Model file for the job. Use its own axes, mm. Face numbers are marked on the shaded views. Round coordinates to 2 decimals unless told otherwise and drop trailing zeros. Order: outer loops, then holes, each group sorted by start corner. A loop starts at its lowest first (then second) coordinate and runs counter-clockwise, first axis right, second up. Notation, with made-up numbers: (-2.75, -21) -> (23.25, -21) arc R21 cw to (23.25, 14) -> close; hole circle Ø10 at (-38.75, -16.75). An arc over 180 degrees is marked (long way). Use CSV: the item, a comma, the result in double quotes.
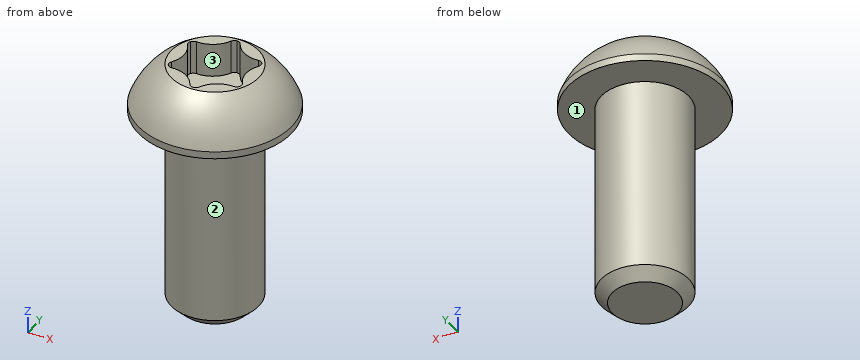
```python
from build123d import *

# Parameters (mm, degrees)
SKETCH12_W         = 14
SKETCH12_H         = 3
CUT_EXTRUDE4_DEPTH = 2.31
CIRPATTERN1_COUNT  = 6
CHAMFER1_SIZE      = 0.75


with BuildPart() as part:
    # Sketch12 → Revolve1 (revolve)
    with BuildSketch(Plane(origin=(0, 0, 0), x_dir=(0, 0, -1), z_dir=(1, 0, 0))):
        with Locations((0, 1.5)):
            Rectangle(SKETCH12_W, SKETCH12_H)
    revolve(axis=Axis((0, 0, -7), (0, 0, 1)))

    # Sketch7 → Revolve2 (revolve)
    with BuildSketch(Plane(origin=(0, 0, 0), x_dir=(0, 0, -1), z_dir=(1, 0, 0)), mode=Mode.PRIVATE) as revolve2_sk:
        with BuildLine():
            Line((-7.495, 5.25), (-7, 5.25))
            Line((-7, 5.25), (-7, 0))
            Line((-7, 0), (-10.3, 0))
            Line((-10.3, 0), (-10.3, 3))
            ThreePointArc((-10.3, 3), (-9.083520981, 4.356906156), (-7.495, 5.25))
        make_face()
    revolve(revolve2_sk.sketch.rotate(Axis((0, 0, 10.3), (0, 0, -1)), 180), axis=Axis((0, 0, 10.3), (0, 0, -1)))

    # Sketch11 → Cut-Extrude4 (cut)
    with BuildSketch(Plane.XY.offset(10.3)):
        with BuildLine():
            Line((0, 0), (-2.430673501, 1.40335))
            ThreePointArc((-2.430673501, 1.40335), (-2.477487573, 1.216409562), (-2.418502657, 1.032945493))
            ThreePointArc((-2.418502657, 1.032945493), (-2.105025, 0), (-2.418502657, -1.032945493))
            ThreePointArc((-2.418502657, -1.032945493), (-2.477487573, -1.216409562), (-2.430673501, -1.40335))
            Line((-2.430673501, -1.40335), (0, 0))
        make_face()
    cut_extrude4 = extrude(amount=-CUT_EXTRUDE4_DEPTH, mode=Mode.SUBTRACT)

    # CirPattern1: Cut-Extrude4 ×6 about axis
    cirpattern1_axis = Axis((0, 0, 0), (0, 0, -1))
    for i in range(1, CIRPATTERN1_COUNT):
        add(cut_extrude4.rotate(cirpattern1_axis, i * 360 / CIRPATTERN1_COUNT), mode=Mode.SUBTRACT)

    # Chamfer1
    chamfer1_edges = [part.edges().sort_by_distance(p)[0] for p in [
        (0, -3, -7),
    ]]
    chamfer(chamfer1_edges, length=CHAMFER1_SIZE)


solid = part.part
```
Q1. Cut at C-C (x = -4.25). Give the cut face in (y, z) (3 decimals), plus the area to 3 significant figures.
From the geometry:
outline,"(-3.082, 7) -> (3.082, 7) -> (3.082, 7.495) arc R3.624 ccw to (-3.082, 7.495) -> close"
area,"10.5 mm²"
Q2. Cut at B-B (z = -5). Give the cut face in (x, y).
From the geometry:
outline,"circle Ø6 at (0, 0)"
Q3. Mould opens along Y. For the marked faces 1, 2 and 3 say: +Y half, -Y half, draft (parallel to the pull), parting line (faces both ways), or undercut.
From the geometry:
face 1,"draft"
face 2,"parting line"
face 3,"undercut"
Q4. Pin check, flat tips, straight feed: pin 1 (1.5 mm diameter, centred on x = 2.5, z = -1, fed in from -Y); pin 2 (5 mm diameter, centred on x = -3.5, y = -4, fed in from -Z); pin 3 (1 mm diameter, centred on y = -2.5, z = 2.5, fed in from +X). Stop position of each tip, or through.
From the geometry:
pin 1,"stops at y = -2.44"
pin 2,"stops at z = -6.43"
pin 3,"stops at x = 2.24"
Q5. Probe line 1 along Z through (x, y) = (-2, 0.5); line 2 along Y through (x, z) = (1.25, 0); line 3 along Y through (x, z) = (2.75, 6). List the from-to ranges inside material, lowest first.
From the geometry:
line 1,"z = -7 to 7.99"
line 2,"y = -2.73 to 2.73"
line 3,"y = -1.2 to 1.2"
Q6. Cut at A-A (y = 0). Give the cut face in (x, z) (3 decimals), plus the area to 3 significant figures.
From the geometry:
outline,"(-5.25, 7) -> (-3, 7) -> (-3, -6.25) -> (-2.25, -7) -> (2.25, -7) -> (3, -6.25) -> (3, 7) -> (5.25, 7) -> (5.25, 7.495) arc R5.585 ccw to (3, 10.3) -> (2.105, 10.3) -> (2.105, 7.99) -> (-2.105, 7.99) -> (-2.105, 10.3) -> (-3, 10.3) arc R5.585 ccw to (-5.25, 7.495) -> close"
area,"103 mm²"
Q7. Cut at D-D (y = -4). Give the cut face in (x, z) (3 decimals).
From the geometry:
outline,"(-3.4, 7) -> (3.4, 7) -> (3.4, 7.495) arc R3.898 ccw to (-3.4, 7.495) -> close"
